from build123d import *

# Parameters (mm, degrees)
SKETCH9_R                       = 9
SKETCH9_R_2                     = 8
BOSS_EXTRUDE1_DEPTH             = 20
SKETCH10_W                      = 4.934959926
SKETCH10_H                      = 0.2
CUT_EXTRUDE1_DEPTH              = 20
SKETCH11_R                      = 6
BOSS_EXTRUDE2_DEPTH             = 100
BOSS_EXTRUDE2_DIRECTION_2_REACH = 23.728
SKETCH12_R                      = 6
BOSS_EXTRUDE3_DEPTH             = 100
BOSS_EXTRUDE3_DIRECTION_2_REACH = 74.864
SKETCH14_R                      = 12.5
CUT_EXTRUDE3_DEPTH              = 82.317279836
CUT_EXTRUDE3_DEPTH_BACK         = 82.317279836
CUT_EXTRUDE4_DEPTH              = 21.0000001


with BuildPart() as part:
    # Sketch9 → Boss-Extrude1 (new body)
    with BuildSketch(Plane.XY):
        Circle(SKETCH9_R)
        Circle(SKETCH9_R_2, mode=Mode.SUBTRACT)
    extrude(amount=BOSS_EXTRUDE1_DEPTH)

    # Sketch10 → Cut-Extrude1 (cut)
    with BuildSketch(Plane.XY.offset(20)):
        with Locations((8, 0)):
            Rectangle(SKETCH10_W, SKETCH10_H)
    extrude(amount=-CUT_EXTRUDE1_DEPTH, mode=Mode.SUBTRACT)

    # Sketch11 → Boss-Extrude2 (add)
    with BuildSketch(Plane(origin=(-6.363961031, 6.363961031, 0), x_dir=(0, 0, -1), z_dir=(-0.707106781, 0.707106781, 0))):
        with Locations((-10, 0)):
            Circle(SKETCH11_R)
    extrude(amount=BOSS_EXTRUDE2_DEPTH)

    # Sketch11 → Boss-Extrude2 direction 2 (add, up to next)
    with BuildSketch(Plane(origin=(-6.363961031, 6.363961031, 0), x_dir=(0, 0, -1), z_dir=(-0.707106781, 0.707106781, 0)), mode=Mode.PRIVATE) as boss_extrude2_direction_2_sk1:
        with Locations((-10, 0)):
            Circle(SKETCH11_R)
    boss_extrude2_direction_2_tool1 = extrude(boss_extrude2_direction_2_sk1.sketch, amount=-BOSS_EXTRUDE2_DIRECTION_2_REACH, mode=Mode.PRIVATE) - part.part
    add(boss_extrude2_direction_2_tool1.solids().sort_by_distance((-6.363961, 6.363961, 10))[0])
    add(boss_extrude2_direction_2_tool1.solids().sort_by_distance((-6.363961, 6.363961, 10))[1])

    # Sketch12 → Boss-Extrude3 (add)
    with BuildSketch(Plane(origin=(6.363961031, 6.363961031, 0), x_dir=(0, 0, -1), z_dir=(0.707106781, 0.707106781, 0))):
        with Locations((-10, 0)):
            Circle(SKETCH12_R)
    extrude(amount=BOSS_EXTRUDE3_DEPTH)

    # Sketch12 → Boss-Extrude3 direction 2 (add, up to next)
    with BuildSketch(Plane(origin=(6.363961031, 6.363961031, 0), x_dir=(0, 0, -1), z_dir=(0.707106781, 0.707106781, 0)), mode=Mode.PRIVATE) as boss_extrude3_direction_2_sk1:
        with Locations((-10, 0)):
            Circle(SKETCH12_R)
    boss_extrude3_direction_2_tool1 = extrude(boss_extrude3_direction_2_sk1.sketch, amount=-BOSS_EXTRUDE3_DIRECTION_2_REACH, mode=Mode.PRIVATE) - part.part
    add(boss_extrude3_direction_2_tool1.solids().sort_by_distance((6.363961, 6.363961, 10))[0])
    add(boss_extrude3_direction_2_tool1.solids().sort_by_distance((6.363961, 6.363961, 10))[1])

    # Sketch14 → Cut-Extrude3 (cut, two sides)
    with BuildSketch(Plane(origin=(0, 0, 0), x_dir=(0, 0, -1), z_dir=(1, 0, 0))) as cut_extrude3_sk:
        with Locations((-10, 79.9)):
            Circle(SKETCH14_R)
    extrude(amount=CUT_EXTRUDE3_DEPTH, mode=Mode.SUBTRACT)
    extrude(cut_extrude3_sk.sketch, amount=-CUT_EXTRUDE3_DEPTH_BACK, mode=Mode.SUBTRACT)

    # Sketch15 → Cut-Extrude4 (cut, through all)
    with BuildSketch(Plane.XY.offset(20)):
        with BuildLine():
            Line((-9, 0), (-109.979142128, 0))
            Line((-109.979142128, 0), (-109.979142128, 78.923804152))
            Line((-109.979142128, 78.923804152), (0, 78.923804152))
            Line((0, 78.923804152), (0, 9))
            ThreePointArc((0, 9), (6.363961031, -6.363961031), (-9, 0))
        make_face()
    extrude(amount=-CUT_EXTRUDE4_DEPTH, mode=Mode.SUBTRACT)


solid = part.part
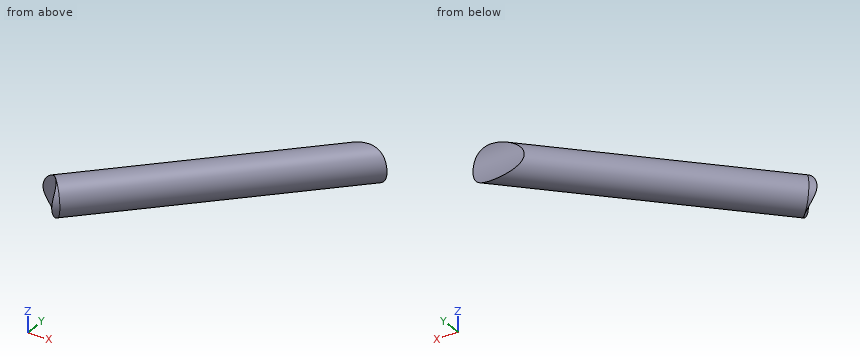
The model under review builds one solid part; all positions refer to its coordinate system, in mm. Coordinates: 2 decimals unless noted, no trailing zeros. Loops run counter-clockwise (first coordinate to the right, second up) from the corner with the lowest first, then second, coordinate; pieces in that order, holes last.
(1) Insertion check: P1, Ø6, axis at y = 21.5, z = 9.5, coming from the +X side; P2, Ø5, axis at y = 30.5, z = 7.5, coming from the +X side; P3, Ø1.5, axis at x = 19, y = 16, coming from the -Z side. Each pin has a flat end and moves straight along its axis. Give the tip position at first contact, or say it passes through.
Determined:
P1: stops at x = 32.97
P2: stops at x = 41.01
P3: stops at z = 4.16
(2) Wall thickness on L1, parallel to Y at x = 40.5, z = 11; L2, parallel to Y at x = 63.5, z = 10.75; L3, parallel to X at y = 36.5, z = 13.5: over which ranges is each line inside the solid? List them lowest first.
Determined:
L1: y = 32.13 to 48.87
L2: y = 55.08 to 67.42
L3: x = 29.61 to 43.39
(3) Consider section A-A, the plane z = 10.5. Give the boundary of the cut face in (x, y), plus the area to 3 significant figures.
Determined:
outline: (0.53, 8.98) arc R9 cw to (8.98, 0.53) - (75.87, 67.41) - (58.95, 67.41) - close
area: 1,040 mm2
(4) Consider section B-B, the plane z = 6. Give the boundary of the cut face in (x, y).
Determined:
outline: (2.36, 8.68) arc R9 cw to (8.68, 2.36) - (74.38, 68.06) - (61.73, 68.06) - close
